from build123d import *

# Parameters (mm, degrees)
BOSS_EXTRUDE1_DEPTH      = 12.7
BOSS_EXTRUDE1_DEPTH_BACK = 12.7
SKETCH1_R                = 2.95
SKETCH1_R_2              = 6.05
CUT_EXTRUDE4_DEPTH       = 86.079315935
CUT_EXTRUDE1_DEPTH       = 81.149563318
FILLET8_R                = 10
CUT_EXTRUDE5_DEPTH       = 81.149563318
FILLET9_R                = 1
LPATTERN1_COUNT          = 3
LPATTERN1_PITCH          = 27
FILLET9_OF_LPATTERN1_R   = 1
CHAMFER2_SIZE            = 0.5
SKETCH8_R                = 4
CUT_EXTRUDE6_DEPTH       = 18
CHAMFER3_SIZE            = 1


with BuildPart() as part:
    # Sketch1 → Boss-Extrude1 (new, two sides: drawn at the far end of the back side and taken through both)
    with BuildSketch(Plane(origin=(0, 0, 0), x_dir=(1, 0, 0), z_dir=(0, 1, 0)).offset(-BOSS_EXTRUDE1_DEPTH_BACK)):
        with BuildLine():
            Line((-67.5, -12.7), (67.5, -12.7))
            ThreePointArc((67.5, -12.7), (80.2, 0), (67.5, 12.7))
            Line((67.5, 12.7), (-67.5, 12.7))
            Line((-67.5, 12.7), (-67.5, -12.7))
        make_face()
        with Locations(Location((67.5, 0, 0), (0, 0, 270))):
            Circle(SKETCH1_R, mode=Mode.SUBTRACT)
        with Locations(Location((42.5, 0, 0), (0, 0, 270))):
            Circle(SKETCH1_R_2, mode=Mode.SUBTRACT)
    extrude(amount=BOSS_EXTRUDE1_DEPTH + BOSS_EXTRUDE1_DEPTH_BACK)

    # Sketch6 → Cut-Extrude4 (cut, through all)
    with BuildSketch(Plane(origin=(0, 12.7, 0), x_dir=(1, 0, 0), z_dir=(0, 1, 0))):
        with BuildLine():
            Line((68.4238, -7.392502524), (43.8082, -10.468577399))
            ThreePointArc((43.8082, -10.468577399), (43.288242133, -10.520512076), (42.766350508, -10.546637256))
            Line((42.766350508, -10.546637256), (-42.5, -12.7))
            Line((-42.5, -12.7), (67.5, -12.7))
            ThreePointArc((67.5, -12.7), (80.2, 0), (67.5, 12.7))
            Line((67.5, 12.7), (-42.5, 12.7))
            Line((-42.5, 12.7), (42.766350508, 10.546637256))
            ThreePointArc((42.766350508, 10.546637256), (43.288242133, 10.520512076), (43.8082, 10.468577399))
            Line((43.8082, 10.468577399), (68.4238, 7.392502524))
            ThreePointArc((68.4238, 7.392502524), (73.085016115, 4.930526848), (74.95, 0))
            ThreePointArc((74.95, 0), (73.085016115, -4.930526848), (68.4238, -7.392502524))
        make_face()
    extrude(amount=-CUT_EXTRUDE4_DEPTH, mode=Mode.SUBTRACT)

    # Sketch2 → Cut-Extrude1 (cut, through all)
    with BuildSketch(Plane(origin=(0, 0, -12.7), x_dir=(-1, 0, 0), z_dir=(0, 0, -1))):
        Polygon((-74.95, 12.7), (43.047588191, 12.7), (5.05, 6), (-74.95, 6), align=None)
        Polygon((-74.95, -12.7), (43.047588191, -12.7), (5.05, -6), (-74.95, -6), align=None)
    extrude(amount=-CUT_EXTRUDE1_DEPTH, mode=Mode.SUBTRACT)

    # Fillet8
    # the kernel refuses this fillet: 10 mm, written as the material it takes off along each edge
    with BuildSketch(Plane(origin=(-127.5, -12.7, 12.7), x_dir=(0, 1, 0), z_dir=(1, 0, 0)), Plane(origin=(16.952411809, -12.7, -12.7), x_dir=(0, 1, 0), z_dir=(-1, 0, 0))) as fillet8_piece_1:
        with BuildLine():
            CenterArc((FILLET8_R, -FILLET8_R), FILLET8_R, 90, 90)
            Line((0, -FILLET8_R), (-FILLET8_R * 0.02, -FILLET8_R))
            Line((-FILLET8_R * 0.02, -FILLET8_R), (-FILLET8_R * 0.02, FILLET8_R * 0.02))
            Line((-FILLET8_R * 0.02, FILLET8_R * 0.02), (FILLET8_R, FILLET8_R * 0.02))
            Line((FILLET8_R, FILLET8_R * 0.02), (FILLET8_R, 0))
        make_face()
    extrude(amount=144.452411809, mode=Mode.SUBTRACT)
    with BuildSketch(Plane(origin=(-127.5, 12.7, 12.7), x_dir=(0, -1, 0), z_dir=(1, 0, 0)), Plane(origin=(16.952411809, 12.7, -12.7), x_dir=(0, -1, 0), z_dir=(-1, 0, 0))) as fillet8_piece_2:
        with BuildLine():
            CenterArc((FILLET8_R, FILLET8_R), FILLET8_R, 180, 90)
            Line((0, FILLET8_R), (-FILLET8_R * 0.02, FILLET8_R))
            Line((-FILLET8_R * 0.02, FILLET8_R), (-FILLET8_R * 0.02, -FILLET8_R * 0.02))
            Line((-FILLET8_R * 0.02, -FILLET8_R * 0.02), (FILLET8_R, -FILLET8_R * 0.02))
            Line((FILLET8_R, -FILLET8_R * 0.02), (FILLET8_R, 0))
        make_face()
    extrude(amount=144.452411809, mode=Mode.SUBTRACT)

    # Sketch7 → Cut-Extrude5 (cut, through all)
    with BuildSketch(Plane(origin=(0, 12.7, 0), x_dir=(1, 0, 0), z_dir=(0, 1, 0))):
        Polygon((-51.5, 8.5), (-51.5, -8.5), (-34.5, -8.5), align=None)
        Polygon((-45.843145751, 8.5), (-28.843145751, -8.5), (-28.843145751, 8.5), align=None)
    cut_extrude5 = extrude(amount=-CUT_EXTRUDE5_DEPTH, mode=Mode.SUBTRACT)

    # Fillet9
    fillet9_edges = [part.edges().sort_by_distance(p)[0] for p in [
        (-28.843145751, 0, -8.5),
        (-45.843145751, 0, -8.5),
        (-28.843145751, 0, 8.5),
        (-34.5, 0, 8.5),
        (-51.5, 0, -8.5),
        (-51.5, 0, 8.5),
    ]]
    fillet(fillet9_edges, radius=FILLET9_R)

    # LPattern1: Cut-Extrude5 ×3
    with Locations(*[(i * LPATTERN1_PITCH, 0, 0) for i in range(1, LPATTERN1_COUNT)]):
        add(cut_extrude5, mode=Mode.SUBTRACT)

    # Fillet9 of LPattern1
    fillet9_of_lpattern1_edges = [part.edges().sort_by_distance(p)[0] for p in [
        (-1.843145751, 0, -8.5),
        (-18.843145751, 0, -8.5),
        (-1.843145751, 0, 8.5),
        (-7.5, 0, 8.5),
        (-24.5, 0, -8.5),
        (-24.5, 0, 8.5),
        (25.156854249, 0, -8.5),
        (8.156854249, 0, -8.5),
        (25.156854249, 0, 8.5),
        (19.5, 0, 8.5),
        (2.5, 0, -8.5),
        (2.5, 0, 8.5),
    ]]
    fillet(fillet9_of_lpattern1_edges, radius=FILLET9_OF_LPATTERN1_R)

    # Chamfer2
    chamfer2_edges = [part.edges().sort_by_distance(p)[0] for p in [
        (18.858175254, -6, 11.150427304),
        (56.116, -6, -8.930539961),
        (18.858175254, -6, -11.150427304),
        (43.288242133, -6, -10.520512076),
        (74.95, -6, 0),
        (43.288242133, -6, 10.520512076),
        (56.116, -6, 8.930539961),
        (56.116, 6, 8.930539961),
        (56.116, 6, -8.930539961),
        (18.858175254, 6, 11.150427304),
        (43.288242133, 6, -10.520512076),
        (18.858175254, 6, -11.150427304),
        (74.95, 6, 0),
        (43.288242133, 6, 10.520512076),
    ]]
    chamfer(chamfer2_edges, length=CHAMFER2_SIZE)

    # Sketch8 → Cut-Extrude6 (cut)
    with BuildSketch(Plane.ZY.offset(67.5)):
        Circle(SKETCH8_R)
    extrude(amount=-CUT_EXTRUDE6_DEPTH, mode=Mode.SUBTRACT)

    # Chamfer3
    chamfer3_edges = [part.edges().sort_by_distance(p)[0] for p in [
        (42.5, 6, -6.05),
    ]]
    chamfer(chamfer3_edges, length=CHAMFER3_SIZE)


solid = part.part
Read the model definition and answer for the solid it produces. Units are mm, in the model's axes. A direction names the side the tool comes from. Give positions to 0.01 mm unless a question says otherwise; leave off trailing zeros. Write each loop counter-clockwise with the first axis right and the second up, starting at its lowest first coordinate (ties: lowest second). Pieces come first, ordered by that corner, then holes. Notation, with made-up numbers: (-21.75, 71) - (26.25, 71) arc R29 ccw to (26.25, 99) - close; hole circle Ø3 at (42.5, -9). An arc over 180 degrees is marked (long way). Return JSON: item names as keys, results as strings.
Q1. A cutting plane is placed at C-C, the plane x = 62. Determine the outline of the cut face in (y, z), and give its area (3 significant figures).
Reply:
{"outline": "(-6, -7.69) - (-5.5, -8.2) - (5.5, -8.2) - (6, -7.69) - (6, 7.69) - (5.5, 8.2) - (-5.5, 8.2) - (-6, 7.69) - close", "area": "196 mm²"}
Q2. For faces 1 (the face through (-67.5, -3, -3)), 2 (the face through (11, 0, 0)), 3 (the face through (-59.612, -3.905, -0.867)), determine the directions among +Z, -Z, +X, -X, +Y, -Y from which every point of the face is accessible in a straight line to the end or side of a thin tool.
Reply:
{"face 1": "+Z, -Z, -X, +Y, -Y", "face 2": "+Y, -Y", "face 3": "-X"}
Q3. For a pull along Z with two mould halves and no side action, classify faces 4 (the face through (-44, 12.7, -2)), 5 (the face through (56.26, -5.75, -8.66)), 6 (the face through (-16, 0, 0)) as released by +Z, released by -Z, zero draft, split by the parting line, or undercut.
Reply:
{"face 4": "zero draft", "face 5": "released by -Z", "face 6": "undercut"}
Q4. A cutting plane is placed at B-B, the plane x = 32. Determine the outline of the cut face in (y, z).
Reply:
{"outline": "(-6, -10.32) - (-5.5, -10.82) - (5.5, -10.82) - (6, -10.32) - (6, 10.32) - (5.5, 10.82) - (-5.5, 10.82) - (-6, 10.32) - close"}
Q5. Consider line 1 along Z through (x, y) = (42.5, -0.5); line 2 along Y through (x, z) = (52, -7); line 3 along Z through (x, y) = (67.5, 0.5). Determine where each line is inside the solid, lowest interval first. Write a range as [from, to].
Reply:
{"line 1": "[-10.55, -6.05], [6.05, 10.55]", "line 2": "[-6, 6]", "line 3": "[-7.51, -2.95], [2.95, 7.51]"}
Q6. Given P1, Ø8, axis at x = -21, y = -8.5, coming from the -Z side; P2, Ø7, axis at y = 1.5, z = 4, coming from the +X side; P3, Ø7, axis at x = 42, z = -5, coming from the -Y side, each flat-ended and moving along its own axis, determine where each tip first touches the part or whether it passes through.
Reply:
{"P1": "z = -12.23", "P2": "x = 74.93", "P3": "y = -6"}
Q7. A cutting plane is placed at A-A, the plane x = -48.5. Determine the outline of the cut face in (y, z).
Reply:
{"outline": "(-12.3, -5.5) arc R10 ccw to (-2.7, -12.7) - (2.7, -12.7) arc R10 ccw to (12.3, -5.5) - close; (-10.85, 8.5) - (10.85, 8.5) arc R10 ccw to (2.7, 12.7) - (-2.7, 12.7) arc R10 ccw to start"}
